```python
from build123d import *

# Parameters (mm, degrees)
SKETCH1_W           = 63.5
SKETCH1_H           = 60.96
BOSS_EXTRUDE1_DEPTH = 40.64
SKETCH2_R           = 24.25
CUT_EXTRUDE1_DEPTH  = 33.02
SKETCH8_W           = 63.5
SKETCH8_H           = 40.64
CUT_EXTRUDE3_DEPTH  = 15.6972
SKETCH16_W          = 25.4
SKETCH16_H          = 40.64
BOSS_EXTRUDE5_DEPTH = 8.89
SKETCH17_R          = 2
CUT_EXTRUDE5_DEPTH  = 79.998181497
SKETCH11_R          = 21.478557246
CUT_EXTRUDE6_DEPTH  = 77.464125575
CHAMFER1_SIZE       = 10


with BuildPart() as part:
    # Sketch1 → Boss-Extrude1 (new body)
    with BuildSketch(Plane.XY):
        Rectangle(SKETCH1_W, SKETCH1_H)
    extrude(amount=BOSS_EXTRUDE1_DEPTH)

    # Sketch2 → Cut-Extrude1 (cut)
    with BuildSketch(Plane.XY.offset(40.64)):
        with Locations((0, -2.08)):
            Circle(SKETCH2_R)
    extrude(amount=-CUT_EXTRUDE1_DEPTH, mode=Mode.SUBTRACT)

    # Sketch8 → Cut-Extrude3 (cut)
    with BuildSketch(Plane(origin=(0, 30.48, 0), x_dir=(1, 0, 0), z_dir=(0, 1, 0))):
        with Locations((0, -20.32)):
            Rectangle(SKETCH8_W, SKETCH8_H)
    extrude(amount=-CUT_EXTRUDE3_DEPTH, mode=Mode.SUBTRACT)

    # Sketch16 → Boss-Extrude5 (add)
    with BuildSketch(Plane.XZ.offset(30.48)):
        with Locations((-44.45, 20.32)):
            Rectangle(SKETCH16_W, SKETCH16_H)
        with Locations((44.45, 20.32)):
            Rectangle(SKETCH16_W, SKETCH16_H)
    extrude(amount=-BOSS_EXTRUDE5_DEPTH)

    # Sketch17 → Cut-Extrude5 (cut, through all)
    with BuildSketch(Plane(origin=(0, -21.59, 0), x_dir=(1, 0, 0), z_dir=(0, 1, 0))):
        with Locations(Location((-52.07, -3.81, 0), (0, 0, 270))):
            Circle(SKETCH17_R)
        with Locations(Location((-52.07, -36.83, 0), (0, 0, 270))):
            Circle(SKETCH17_R)
        with Locations(Location((52.07, -3.81, 0), (0, 0, 270))):
            Circle(SKETCH17_R)
        with Locations(Location((52.07, -36.83, 0), (0, 0, 270))):
            Circle(SKETCH17_R)
    extrude(amount=-CUT_EXTRUDE5_DEPTH, mode=Mode.SUBTRACT)

    # Sketch11 → Cut-Extrude6 (cut, through all)
    with BuildSketch(Plane(origin=(0, 0, 0), x_dir=(-1, 0, 0), z_dir=(0, 0, -1))):
        Circle(SKETCH11_R)
    extrude(amount=-CUT_EXTRUDE6_DEPTH, mode=Mode.SUBTRACT)

    # Chamfer1
    chamfer1_edges = [part.edges().sort_by_distance(p)[0] for p in [
        (-31.75, -21.59, 20.32),
        (31.75, -21.59, 20.32),
    ]]
    chamfer(chamfer1_edges, length=CHAMFER1_SIZE)


solid = part.part
```
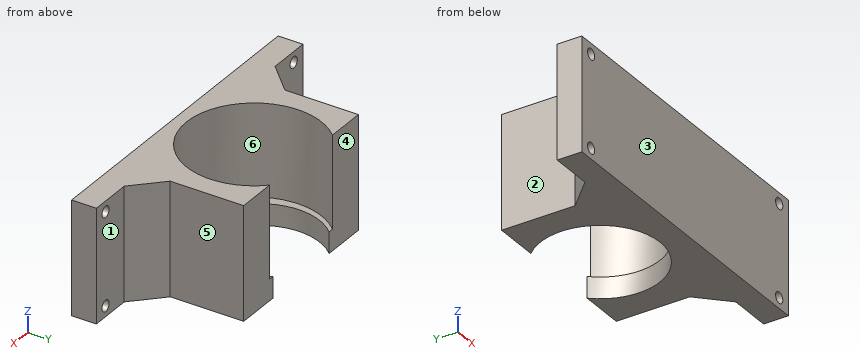
The listing builds one solid part. Answer for the finished solid, in the listing's coordinates (mm). Face numbers are marked on the shaded views. A direction names the side the tool comes from. Coordinates: 2 decimals unless noted, no trailing zeros. Loops run counter-clockwise (first coordinate to the right, second up) from the corner with the lowest first, then second, coordinate; pieces in that order, holes last. Notation, with made-up numbers: (-16.5, -7.5) -> (1.5, -7.5) arc R14 ccw to (1.5, 19.5) -> close; hole circle Ø1 at (80.25, 53.25). An arc over 180 degrees is marked (long way). Use one line per item in the form item = value. Start each with the question number.
Item 1: The mould has two halves that part along Y. Classify the marked faces 4, 5 and 6: released by +Y, released by -Y, zero draft, split by the parting line, or undercut.
Item 2: The part is cut by section C-C on x = -52.07. Determine the outline of the cut face in (y, z), then the cut area to 3 significant figures.
Item 3: The part is cut by section A-A on z = 3.81. Determine the outline of the cut face in (x, y), then the cut area to 3 significant figures.
Item 4: Consider L1, parallel to Z at x = 52, y = -27; L2, parallel to X at y = -2.08, z = 29.5; L3, parallel to X at y = 0, z = 2.25. Determine where each line is inside the solid, lowest interval first. Write a range as [from, to].
Item 5: The part is cut by section D-D on y = -7. Determine the outline of the cut face in (x, z), then the cut area to 3 significant figures.
Item 6: The part is cut by section B-B on y = 0. Determine the outline of the cut face in (x, z), then the cut area to 3 significant figures.
Item 7: Flat-ended cylindrical pins translate along their axes: pin 1 Ø1 at (y, z) = (-8.5, 31.5) entering from +X; pin 2 Ø10 at (y, z) = (-15, 36) entering from -X; pin 3 Ø17 at (x, z) = (48, 20) entering from +Y. Find the tip coordinate at first contact, or state that the pin passes through.
Item 8: A tool of negligible diameter and unlimited length cuts with its end or side. For the marked faces 1, 2 and 3, from which of +Z, -Z, +X, -X, +Y, -Y can it reach the whole face along a straight path? Write none if from no direction.
Answer key:
q1.face_4 = released by +Y
q1.face_5 = zero draft
q1.face_6 = undercut
q2.outline = (-30.48, 0) -> (-21.59, 0) -> (-21.59, 1.81) -> (-30.48, 1.81) -> close; (-30.48, 5.81) -> (-21.59, 5.81) -> (-21.59, 34.83) -> (-30.48, 34.83) -> close; (-30.48, 38.83) -> (-21.59, 38.83) -> (-21.59, 40.64) -> (-30.48, 40.64) -> close
q2.area = 290 mm2
q3.outline = (-57.15, -30.48) -> (-54.07, -30.48) -> (-54.07, -21.59) -> (-57.15, -21.59) -> close; (-50.07, -30.48) -> (50.07, -30.48) -> (50.07, -21.59) -> (41.75, -21.59) -> (31.75, -11.59) -> (31.75, 14.78) -> (15.58, 14.78) arc R21.48 cw (long way) to (-15.58, 14.78) -> (-31.75, 14.78) -> (-31.75, -11.59) -> (-41.75, -21.59) -> (-50.07, -21.59) -> close; (54.07, -30.48) -> (57.15, -30.48) -> (57.15, -21.59) -> (54.07, -21.59) -> close
q3.area = 2,050 mm2
q4.L1 = [0, 1.81], [5.81, 34.83], [38.83, 40.64]
q4.L2 = [-31.75, -24.25], [24.25, 31.75]
q4.L3 = [-31.75, -21.48], [21.48, 31.75]
q5.outline = (-31.75, 0) -> (-20.31, 0) -> (-20.31, 7.62) -> (-23.75, 7.62) -> (-23.75, 40.64) -> (-31.75, 40.64) -> close; (20.31, 0) -> (31.75, 0) -> (31.75, 40.64) -> (23.75, 40.64) -> (23.75, 7.62) -> (20.31, 7.62) -> close
q5.area = 703 mm2
q6.outline = (-31.75, 0) -> (-21.48, 0) -> (-21.48, 7.62) -> (-24.16, 7.62) -> (-24.16, 40.64) -> (-31.75, 40.64) -> close; (21.48, 0) -> (31.75, 0) -> (31.75, 40.64) -> (24.16, 40.64) -> (24.16, 7.62) -> (21.48, 7.62) -> close
q6.area = 658 mm2
q7.pin_1 = 31.75
q7.pin_2 = -40.16
q7.pin_3 = -19.34
q8.face_1 = +Z, -Z, +X, +Y
q8.face_2 = +Z, -Z, -X, +Y
q8.face_3 = +Z, -Z, +X, -X, -Y
